Could you check a few things on this model? Use its own coordinates, in mm. Round coordinates to 2 decimals unless told otherwise and drop trailing zeros. Loops run counter-clockwise (first coordinate to the right, second up) from the corner with the lowest first, then second, coordinate; pieces in that order, holes last. Notation, with made-up numbers: (25, 9.25) -> (39, 9.25) arc R22 ccw to (39, 33.25) -> close; hole circle Ø4 at (-6.5, 18). An arc over 180 degrees is marked (long way). Put each result on its own line as item: value. Start each with the question number.
1. Imagine slicing it at C-C, the plane z = -36. Please give me the cut outline in (x, y), and give its area (3 significant figures).
2. Imagine slicing it at B-B, the plane y = 6. Please give me the cut outline in (x, z), and give its area (3 significant figures).
3. I need wall thicknesses on line 1 (Y direction, x = -6.75, z = -6.5); line 2 (Y direction, x = -2.5, z = -3.5); line 3 (Y direction, x = -9, z = -31.5). Which ranges of each line are inside material? Lowest first, please. Write a range as [from, to].
4. Imagine slicing it at D-D, the plane z = -19.5. Please give me the cut outline in (x, y), and give its area (3 significant figures).
5. Imagine slicing it at A-A, the plane x = -5. Please give me the cut outline in (y, z), and give its area (3 significant figures).
6. I'm going to push flat-ended pins straight in: P1, Ø3, axis at x = -1, z = -15.5, coming from the +Y side; P2, Ø2, axis at y = 2.5, z = -13, coming from the +X side. Where does each tip first touch, or does it pass through?
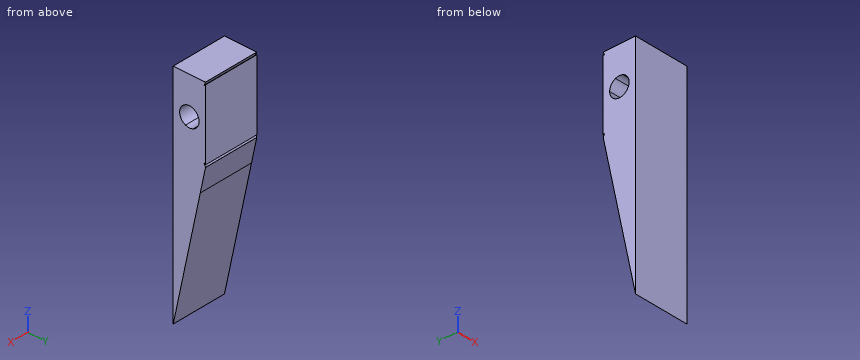
```python
from build123d import *

# Parameters (mm, degrees)
F1_DEPTH = 11.43


with BuildPart() as f1:
    # F0 (on Right) → F1 (new body)
    with BuildSketch(Plane.YZ):
        Polygon((3.3542175311, -1.5767664933), (1.4732253194, 2.7673263745), (1.4732253194, -3.1085191088), align=None)
        Polygon((7.7828650435, 2.029623989), (8.1059029485, 2.775669959), (1.4732253194, 2.775669959), (1.4732253194, 2.7673263745), (3.3542175311, -1.5767664933), align=None)
        with BuildLine():
            Line((8.1059029485, -12.0676500307), (8.1059029485, 2.2926841722))
            Line((8.1059029485, 2.2926841722), (7.7828650435, 2.029623989))
            Line((7.7828650435, 2.029623989), (5.5800336964, -3.0577463276))
            ThreePointArc((5.5800336964, -3.0577463276), (6.4543945145, -3.7929697506), (6.7816577479, -4.8874829292))
            ThreePointArc((6.7816577479, -4.8874829292), (6.4543945145, -5.9819961078), (5.5800336964, -6.7172195309))
            Line((5.5800336964, -6.7172195309), (7.7828650435, -11.8045898475))
            Line((7.7828650435, -11.8045898475), (8.1059029485, -12.0676500307))
        make_face()
        Polygon((1.4732253194, -12.5422922329), (8.1022901764, -12.5422922329), (7.7828650435, -11.8045898475), (3.3542175311, -8.1981993651), align=None)
        Polygon((3.3542175311, -8.1981993651), (1.4732253194, -6.6664467497), (1.4732253194, -12.5422922329), align=None)
        with BuildLine():
            Line((3.3542175311, -8.1981993651), (7.7828650435, -11.8045898475))
            Line((7.7828650435, -11.8045898475), (5.5800336964, -6.7172195309))
            ThreePointArc((5.5800336964, -6.7172195309), (4.7877577479, -6.8813829292), (3.9954817993, -6.7172195309))
            Line((3.9954817993, -6.7172195309), (3.3542175311, -8.1981993651))
        make_face()
        with BuildLine():
            Line((1.4732253194, -3.1085191088), (1.4732253194, -6.6664467497))
            Line((1.4732253194, -6.6664467497), (3.3542175311, -8.1981993651))
            Line((3.3542175311, -8.1981993651), (3.9954817993, -6.7172195309))
            ThreePointArc((3.9954817993, -6.7172195309), (2.7938577479, -4.8874829292), (3.9954817993, -3.0577463276))
            Line((3.9954817993, -3.0577463276), (3.3542175311, -1.5767664933))
            Line((3.3542175311, -1.5767664933), (1.4732253194, -3.1085191088))
        make_face()
        with BuildLine():
            Line((5.5800336964, -3.0577463276), (7.7828650435, 2.029623989))
            Line((7.7828650435, 2.029623989), (3.3542175311, -1.5767664933))
            Line((3.3542175311, -1.5767664933), (3.9954817993, -3.0577463276))
            ThreePointArc((3.9954817993, -3.0577463276), (4.7877577479, -2.8935829292), (5.5800336964, -3.0577463276))
        make_face()
        Polygon((1.4732253194, -43.5194037855), (7.0256497619, -17.5874829292), (1.4732253194, -17.5874829292), align=None)
        Polygon((1.4732253194, -17.5874829292), (7.0256497619, -17.5874829292), (8.1047075663, -12.5478751196), (8.1022901764, -12.5422922329), (1.4732253194, -12.5422922329), align=None)
    extrude(amount=-F1_DEPTH)


solid = f1.part
```
Entries:
1. outline: (-11.43, 1.47) -> (0, 1.47) -> (0, 3.08) -> (-11.43, 3.08) -> close
1. area: 18.4 mm^2
2. outline: (-11.43, -22.38) -> (0, -22.38) -> (0, -6.47) -> (-11.43, -6.47) -> close; (-11.43, -3.3) -> (0, -3.3) -> (0, 2.78) -> (-11.43, 2.78) -> close
2. area: 251 mm^2
3. line 1: [1.47, 3.61], [5.96, 8.11]
3. line 2: [1.47, 3.36], [6.22, 8.11]
3. line 3: [1.47, 4.05]
4. outline: (-11.43, 1.47) -> (0, 1.47) -> (0, 6.62) -> (-11.43, 6.62) -> close
4. area: 58.8 mm^2
5. outline: (1.47, -43.52) -> (8.1, -12.55) -> (7.78, -11.8) -> (8.11, -12.07) -> (8.11, 2.29) -> (7.78, 2.03) -> (8.11, 2.78) -> (1.47, 2.78) -> close; hole circle Ø3.99 at (4.79, -4.89)
5. area: 192 mm^2
6. P1: y = 7.79
6. P2: x = 0
